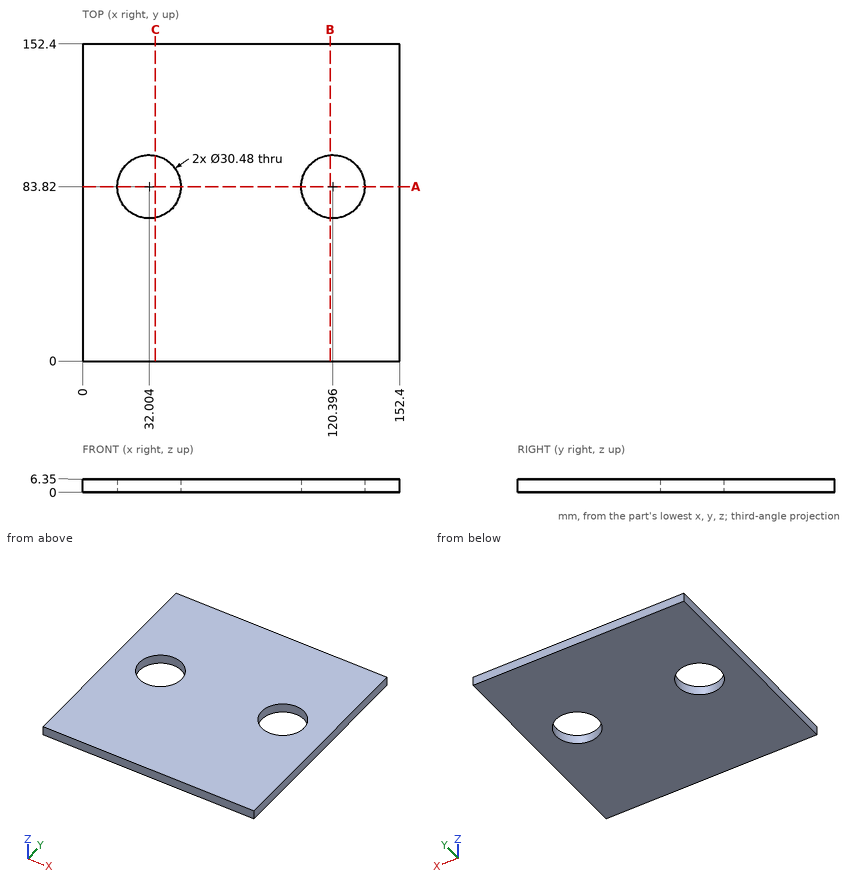
Source: three-view drawing plus pictorial views. Frame: mm from the lowest corner of the part. Round coordinates to 2 decimals unless told otherwise and drop trailing zeros. Write each loop counter-clockwise with the first axis right and the second up, starting at its lowest first coordinate (ties: lowest second). Pieces come first, ordered by that corner, then holes. Notation, with made-up numbers: M 19.5,76.25 L 60.5,76.25 A22 cw 60.5,88.25 Z; hole C -4,60.5 d1. An arc over 180 degrees is marked long. Use CSV: the item, a comma, the result in double quotes. Start each with the question number.
Q1. Cut plane B-B on x = 119. Output: boundary loops of the cut face in (y, z), plus the area to 3 significant figures.
Q2. Cut plane C-C on x = 35. Output: boundary loops of the cut face in (y, z).
Q3. Cut plane A-A on y = 83.82. Output: boundary loops of the cut face in (x, z).
Q4. Line query: line 1 (Y direction, x = 130, z = 2.75); line 2 (Y direction, x = 132.5, z = 5.5). Output: solid intervals per line, ascending. Write a range as from..to.
Q5. First-contact query: P1, Ø24.5, axis at x = 32.004, y = 83.82, coming from the +Z side. Flat tip, straight axial feed; report the tip coordinate or a pass-through.
Results found:
1,outline,"M 0,0 L 68.64,0 L 68.64,6.35 L 0,6.35 Z; M 99,0 L 152.4,0 L 152.4,6.35 L 99,6.35 Z"
1,area,"775 mm^2"
2,outline,"M 0,0 L 68.88,0 L 68.88,6.35 L 0,6.35 Z; M 98.76,0 L 152.4,0 L 152.4,6.35 L 98.76,6.35 Z"
3,outline,"M 0,0 L 16.76,0 L 16.76,6.35 L 0,6.35 Z; M 47.24,0 L 105.16,0 L 105.16,6.35 L 47.24,6.35 Z; M 135.64,0 L 152.4,0 L 152.4,6.35 L 135.64,6.35 Z"
4,line 1,"0..71.99, 95.65..152.4"
4,line 2,"0..74.56, 93.08..152.4"
5,P1,"through"
